Read the model definition and answer for the solid it produces. Units are mm, in the model's axes. A direction names the side the tool comes from. Give positions to 0.01 mm unless a question says otherwise; leave off trailing zeros. Order: outer loops, then holes, each group sorted by start corner. A loop starts at its lowest first (then second) coordinate and runs counter-clockwise, first axis right, second up. Notation, with made-up numbers: (34.25, 79.25) - (68.25, 79.25) arc R26 ccw to (68.25, 97.25) - close; hole circle Ø2 at (1, 78.5). An arc over 180 degrees is marked (long way). Use a Markdown table: item, result. Add a question column.
1. Flat-ended cylindrical pins translate along their axes: P1, Ø10, axis at x = 53, y = 58.5, coming from the +Z side; P2, Ø12, axis at x = 8, y = 32.5, coming from the +Z side; P3, Ø8, axis at x = -37.5, y = 28.5, coming from the +Z side; P4, Ø4, axis at x = 48.26, z = 0, coming from the -Y side. Find the tip coordinate at first contact, or state that the pin passes through.
2. A cutting plane is placed at D-D on x = 48.26. Determine the outline of the cut face in (y, z).
3. A cutting plane is placed at C-C on y = 10. Determine the outline of the cut face in (x, z).
4. A cutting plane is placed at B-B on z = 0. Determine the outline of the cut face in (x, y).
5. Consider L1, parallel to X at y = -3, z = 0; L2, parallel to X at y = 49.5, z = 0; L3, parallel to Y at x = 42.5, z = -44. Determine where each line is inside the solid, lowest interval first.
6. Which of the six approach directions +Z, -Z, +X, -X, +Y, -Y give full straight-line access (tool end or side, diameter ignored) to faces 1 (the flat face through (1, 0, 1)), 2 (the cylindrical face through (1.015, -2.576, 45.038))?
7. A cutting plane is placed at A-A on x = 0. Determine the outline of the cut face in (y, z), and give its area (3 significant figures).
```python
from build123d import *

# Parameters (mm, degrees)
SKETCH1_R           = 73.66
SKETCH1_R_2         = 68.58
BOSS_EXTRUDE1_DEPTH = 104.14
BOSS_EXTRUDE2_START = 5.08
SKETCH2_R           = 73.66
SKETCH2_R_2         = 3.3782
BOSS_EXTRUDE2_DEPTH = 5.08


with BuildPart() as part:
    # Sketch1 → Boss-Extrude1 (new body)
    with BuildSketch(Plane(origin=(0, 0, 0), x_dir=(1, 0, 0), z_dir=(0, 1, 0))):
        with Locations(Location((0, 0, 0), (0, 0, 270))):
            Circle(SKETCH1_R)
        with Locations(Location((0, 0, 0), (0, 0, 270))):
            Circle(SKETCH1_R_2, mode=Mode.SUBTRACT)
    extrude(amount=BOSS_EXTRUDE1_DEPTH)

    # Sketch2 → Boss-Extrude2 (add)
    with BuildSketch(Plane.XZ.offset(BOSS_EXTRUDE2_START)):
        with Locations(Location((0, 0, 0), (0, 0, 270))):
            Circle(SKETCH2_R)
        with Locations(Location((0, 48.26, 0), (0, 0, 270))):
            Circle(SKETCH2_R_2, mode=Mode.SUBTRACT)
        with Locations(Location((48.26, 0, 0), (0, 0, 270))):
            Circle(SKETCH2_R_2, mode=Mode.SUBTRACT)
        with Locations(Location((0, -48.26, 0), (0, 0, 270))):
            Circle(SKETCH2_R_2, mode=Mode.SUBTRACT)
        with Locations(Location((-48.26, 0, 0), (0, 0, 270))):
            Circle(SKETCH2_R_2, mode=Mode.SUBTRACT)
    extrude(amount=-BOSS_EXTRUDE2_DEPTH)


solid = part.part
```
Output values:
| question | item | result |
|---|---|---|
| 1 | P1 | z = 55.87 |
| 1 | P2 | z = 73.63 |
| 1 | P3 | z = 65.6 |
| 1 | P4 | through |
| 2 | outline | (-5.08, -55.65) - (104.14, -55.65) - (104.14, -48.73) - (0, -48.73) - (0, -3.38) - (-5.08, -3.38) - close; (-5.08, 3.38) - (0, 3.38) - (0, 48.73) - (104.14, 48.73) - (104.14, 55.65) - (-5.08, 55.65) - close |
| 3 | outline | circle Ø147.32 at (0, 0); hole circle Ø137.16 at (0, 0) |
| 4 | outline | (-73.66, -5.08) - (-51.64, -5.08) - (-51.64, 0) - (-68.58, 0) - (-68.58, 104.14) - (-73.66, 104.14) - close; (-44.88, -5.08) - (44.88, -5.08) - (44.88, 0) - (-44.88, 0) - close; (51.64, -5.08) - (73.66, -5.08) - (73.66, 104.14) - (68.58, 104.14) - (68.58, 0) - (51.64, 0) - close |
| 5 | L1 | -73.66 to -51.64, -44.88 to 44.88, 51.64 to 73.66 |
| 5 | L2 | -73.66 to -68.58, 68.58 to 73.66 |
| 5 | L3 | -5.08 to 0 |
| 6 | face 1 | +Y |
| 6 | face 2 | +Y, -Y |
| 7 | outline | (-5.08, -73.66) - (104.14, -73.66) - (104.14, -68.58) - (0, -68.58) - (0, -51.64) - (-5.08, -51.64) - close; (-5.08, -44.88) - (0, -44.88) - (0, 44.88) - (-5.08, 44.88) - close; (-5.08, 51.64) - (0, 51.64) - (0, 68.58) - (104.14, 68.58) - (104.14, 73.66) - (-5.08, 73.66) - close |
| 7 | area | 1,740 mm² |
